```python
from build123d import *

# Parameters (mm, degrees)
PAD_DEPTH = 12.8


with BuildPart() as part:
    # Sketch → Pad (new body)
    with BuildSketch(Plane.XY):
        with BuildLine():
            ThreePointArc((-24.295471, 26.987861), (-22.525854, 20.33745), (-20.005224, 13.933863))
            ThreePointArc((-20.005224, 13.933863), (-14.526243, 3.599075), (-7.945722, -6.071697))
            ThreePointArc((-7.945722, -6.071697), (0, -10), (7.945722, -6.071697))
            ThreePointArc((7.945722, -6.071697), (14.526243, 3.599075), (20.005224, 13.933863))
            ThreePointArc((20.005224, 13.933863), (22.525853, 20.337445), (24.295472, 26.98785))
            ThreePointArc((24.295472, 26.98785), (22.666335, 34.771566), (15.872783, 38.905324))
            ThreePointArc((15.872783, 38.905324), (7.955243, 39.726006), (0, 40))
            ThreePointArc((0, 40), (-7.955239, 39.726008), (-15.872775, 38.905329))
            ThreePointArc((-15.872775, 38.905329), (-22.666329, 34.771574), (-24.295471, 26.987861))
        make_face()
        with BuildLine():
            Line((3.631735, 2.323545), (14.769834, 26.452216))
            ThreePointArc((14.769834, 26.452216), (14.60588, 28.847319), (12.5, 30))
            Line((-12.5, 30), (12.5, 30))
            ThreePointArc((-12.5, 30), (-14.60588, 28.847319), (-14.769834, 26.452216))
            Line((-3.631735, 2.323545), (-14.769834, 26.452216))
            ThreePointArc((-3.631735, 2.323545), (0, 0), (3.631735, 2.323545))
        make_face(mode=Mode.SUBTRACT)
    extrude(amount=PAD_DEPTH)


solid = part.part
```
For this review, take the finished solid that the model builds, in its own axes (mm). A direction names the side the tool comes from. Give positions to 0.01 mm unless a question says otherwise; leave off trailing zeros. Write each loop counter-clockwise with the first axis right and the second up, starting at its lowest first coordinate (ties: lowest second). Pieces come first, ordered by that corner, then holes. Notation, with made-up numbers: M 79.5,56.25 L 106.5,56.25 A15 cw 106.5,60.25 Z; hole C 30.25,48 d1. An arc over 180 degrees is marked long. Answer as a JSON object with one key per item and string values. Group by question number.
Item 1: Tool access review of faces 4 (the cylindrical face through (8.07, 39.72, 6.31)), 5 (the cylindrical face through (-14.587, 28.877, 6.31)): name each direction out of +Z, -Z, +X, -X, +Y, -Y from which nothing blocks a thin tool from reaching the whole face with its end or side.
Item 2: Consider section C-C on y = 21.5. Write out the cut boundary in (x, z), plus the area to 3 significant figures.
Item 3: For probe 1 along Y at (x, z) = (-2, 10.25); probe 2 along X at (y, z) = (4, 1.5); probe 3 along X at (y, z) = (12, 3.75), list the stretches that pass through material, from the lowest coordinate up. Write a range as [from, to].
Item 4: Consider section A-A on x = -3. Write out the cut boundary in (y, z).
Item 5: Draft analysis for pull direction X (two halves, no side actions). For faces 1 (the flat face through (9.123, 14.219, 6.31)), 2 (the flat face through (11, 15, 0)), 3 (the cylindrical face through (0, -10, 6)), state which applies: +X half, -X half, draft (parallel to the pull), parting line (faces both ways), or undercut.
Item 6: Consider section B-B on z = 8. Write out the cut boundary in (x, y).
Item 7: For pin 1 Ø6.5 at (x, z) = (5, 5) entering from -Y; pin 2 Ø3 at (y, z) = (35, 5.5) entering from +X; pin 3 Ø5 at (y, z) = (15.5, 4) entering from +X, all flat-tipped, find the tip position at first contact; note any pin that passes through.
Item 8: Consider section D-D on y = 35. Write out the cut boundary in (x, z).
Check result:
{
 "1": {"face 4": "+Z, -Z, +X, +Y", "face 5": "+Z, -Z"},
 "2": {"outline": "M -22.89,0 L -12.48,0 L -12.48,12.8 L -22.89,12.8 Z; M 12.48,0 L 22.89,0 L 22.89,12.8 L 12.48,12.8 Z", "area": "267 mm^2"},
 "3": {"probe 1": "y = [-9.8, 0.54], [30, 39.98]", "probe 2": "x = [-14.77, -4.41], [4.41, 14.77]", "probe 3": "x = [-19.09, -8.1], [8.1, 19.09]"},
 "4": {"outline": "M -9.54,0 L 1.35,0 L 1.35,12.8 L -9.54,12.8 Z; M 30,0 L 39.96,0 L 39.96,12.8 L 30,12.8 Z"},
 "5": {"face 1": "undercut", "face 2": "draft", "face 3": "parting line"},
 "6": {"outline": "M -24.3,26.99 A59.91 ccw -20.01,13.93 A106.38 ccw -7.95,-6.07 A10 ccw 7.95,-6.07 A106.38 ccw 20.01,13.93 A59.91 ccw 24.3,26.99 A10 ccw 15.87,38.91 A115.63 ccw 0,40 A115.63 ccw -15.87,38.91 A10 ccw Z; hole M -14.77,26.45 L -3.63,2.32 A4 ccw 3.63,2.32 L 14.77,26.45 A2.5 ccw 12.5,30 L -12.5,30 A2.5 ccw Z"},
 "7": {"pin 1": "stops at y = -9.85", "pin 2": "stops at x = 23.43", "pin 3": "stops at x = 21.7"},
 "8": {"outline": "M -22.5,0 L 22.5,0 L 22.5,12.8 L -22.5,12.8 Z"}
}
